Geometry: final body of the model. Coordinates: model frame, mm. Give positions to 0.01 mm unless a question says otherwise; leave off trailing zeros. Write each loop counter-clockwise with the first axis right and the second up, starting at its lowest first coordinate (ties: lowest second). Pieces come first, ordered by that corner, then holes.
Q1. Cut plane B-B on x = -64. Count the separate pieces of the cut face and the enclosed holes in it, plus the area to 3 significant figures.
Q2. Line query: L1, parallel to Y at x = -64, z = 5; L2, parallel to X at y = -174, z = 4.5; L3, parallel to X at y = -361.5, z = 7.75. Output: solid intervals per line, ascending.
Q3. Pin query (flat end, axial travel): pin 1 (8 mm diameter, centred on x = -13, y = -416.06, fed in from +Z). Return the tip coordinate at first contact, or that it passes through.
Q4. Cut plane A-A on x = -115.5. Return the cut outline in (y, z).
Q5. Cut plane C-C on y = -180.5. Return the cut outline in (x, z).
Q6. Draft query along Y for faces 1 (the face through (-34.045, -126.664, 4.056)), 2 (the face through (-65, -260, 0)), 3 (the face through (-10.69, -280.18, 4.06)), 4 (the face through (-113.568, -201.389, 3.944)). Return one class per face: pulls with the +Y half, pulls with the -Y half, needs draft (parallel to the pull), parting line crosses it, or undercut.
Autodesk Inventor part; units mm, degrees
ref_plane "Work Plane1" through (0, 0, 0) normal (0, 0, 1) x (1, 0, 0)
ref_plane "YZ Plane" through (0, 0, 0) normal (1, 0, 0) x (0, 1, 0)
ref_plane "XZ Plane" through (0, 0, 0) normal (0, 1, 0) x (-1, 0, 0)
ref_plane "Work Plane1" through (0, 0, 0) normal (0, 0, 1) x (1, 0, 0)
sketch "Sketch1" plane through (0, 0, 0) normal (0, 0, 1) x (1, 0, 0)
  line L0 (-65.5, -425.0611) -> (-65.5, -432.1593)
  line L1 (-120, -425.0611) -> (-65.5, -425.0611)
  ellipse E0 centre (-120, -417.963) end of major axis (-120, -425.0611) minor radius 4 (-124, -417.963) -> (-120, -425.0611) ccw
  line L2 (-124, -275.99) -> (-124, -417.963)
  ellipse E1 centre (-120, -275.99) end of major axis (-120, -268.8918) minor radius 4 (-123.8796, -274.2613) -> (-124, -275.99) ccw
  line L3 (-103.5409, -130.5299) -> (-123.8796, -274.2613)
  ellipse E2 centre (-99.6613, -132.2586) end of major axis (-99.6613, -125.1604) minor radius 4 (-103.1868, -128.9053) -> (-103.5409, -130.5299) ccw
  line L4 (-67.5255, -10.843) -> (-103.1868, -128.9053)
  ellipse E3 centre (-64, -14.1963) end of major axis (-64, -7.0982) minor radius 4 (-60.4745, -10.843) -> (-67.5255, -10.843) ccw
  line L5 (-24.8132, -128.9053) -> (-60.4745, -10.843)
  ellipse E4 centre (-28.3387, -132.2586) end of major axis (-28.3387, -125.1604) minor radius 4 (-24.4591, -130.5299) -> (-24.8132, -128.9053) ccw
  line L6 (-4.1204, -274.2613) -> (-24.4591, -130.5299)
  ellipse E5 centre (-8, -275.99) end of major axis (-8, -268.8918) minor radius 4 (-4, -275.99) -> (-4.1204, -274.2613) ccw
  line L7 (-4, -417.963) -> (-4, -275.99)
  ellipse E6 centre (-8, -417.963) end of major axis (-8, -425.0611) minor radius 4 (-8, -425.0611) -> (-4, -417.963) ccw
  line L8 (-62.5, -425.0611) -> (-8, -425.0611)
  line L9 (-62.5, -432.1593) -> (-62.5, -425.0611)
  line L10 (-8, -432.1593) -> (-62.5, -432.1593)
  ellipse E7 centre (-8, -417.963) end of major axis (-8, -432.1593) minor radius 8 (-8, -432.1593) -> (0, -417.963) ccw
  line L11 (0, -275.99) -> (0, -417.963)
  ellipse E8 centre (-8, -275.99) end of major axis (-8, -261.7937) minor radius 8 (0, -275.99) -> (-0.2409, -272.5326) ccw
  line L12 (-20.5796, -128.8012) -> (-0.2409, -272.5326)
  ellipse E9 centre (-28.3387, -132.2586) end of major axis (-28.3387, -118.0623) minor radius 8 (-20.5796, -128.8012) -> (-21.2877, -125.5519) ccw
  line L13 (-56.949, -7.4896) -> (-21.2877, -125.5519)
  ellipse E10 centre (-64, -14.1963) end of major axis (-64, 0) minor radius 8 (-56.949, -7.4896) -> (-71.051, -7.4896) ccw
  line L14 (-106.7123, -125.5519) -> (-71.051, -7.4896)
  ellipse E11 centre (-99.6613, -132.2586) end of major axis (-99.6613, -118.0623) minor radius 8 (-106.7123, -125.5519) -> (-107.4204, -128.8012) ccw
  line L15 (-127.7591, -272.5326) -> (-107.4204, -128.8012)
  ellipse E12 centre (-120, -275.99) end of major axis (-120, -261.7937) minor radius 8 (-127.7591, -272.5326) -> (-128, -275.99) ccw
  line L16 (-128, -417.963) -> (-128, -275.99)
  ellipse E13 centre (-120, -417.963) end of major axis (-120, -432.1593) minor radius 8 (-128, -417.963) -> (-120, -432.1593) ccw
  line L17 (-65.5, -432.1593) -> (-120, -432.1593)
  line L18 (-62.5, -425.0611) -> (-65.5, -425.0611)
  point P0 (0, 0)
extrude "Plate1" add sketch "Sketch1" along normal blind 8 contours L1 E0 L2 E1 L3 E2 L4 E3 L5 E4 L6 E5 L7 E6 L8 L18
sketch "Sketch2" plane through (0, 0, 8) normal (0, 0, 1) x (1, 0, 0)
  line L0 (-8, -425.0611) -> (-120, -425.0611)
  ellipse E0 centre (-8, -417.963) end of major axis (-8, -425.0611) minor radius 4 (-8, -425.0611) -> (-4, -417.963) ccw
  line L1 (-4, -275.99) -> (-4, -417.963)
  ellipse E1 centre (-8, -275.99) end of major axis (-8, -268.8918) minor radius 4 (-4, -275.99) -> (-4.1204, -274.2613) ccw
  line L2 (-24.4591, -130.5299) -> (-4.1204, -274.2613)
  ellipse E2 centre (-28.3387, -132.2586) end of major axis (-28.3387, -125.1604) minor radius 4 (-24.4591, -130.5299) -> (-24.8132, -128.9053) ccw
  line L3 (-60.4745, -10.843) -> (-24.8132, -128.9053)
  ellipse E3 centre (-64, -14.1963) end of major axis (-64, -7.0982) minor radius 4 (-60.4745, -10.843) -> (-67.5255, -10.843) ccw
  line L4 (-103.1868, -128.9053) -> (-67.5255, -10.843)
  ellipse E4 centre (-99.6613, -132.2586) end of major axis (-99.6613, -125.1604) minor radius 4 (-103.1868, -128.9053) -> (-103.5409, -130.5299) ccw
  line L5 (-123.8796, -274.2613) -> (-103.5409, -130.5299)
  ellipse E5 centre (-120, -275.99) end of major axis (-120, -268.8918) minor radius 4 (-123.8796, -274.2613) -> (-124, -275.99) ccw
  line L6 (-124, -417.963) -> (-124, -275.99)
  ellipse E6 centre (-120, -417.963) end of major axis (-120, -425.0611) minor radius 4 (-124, -417.963) -> (-120, -425.0611) ccw
  line L7 (-64, -470.7435) -> (-64, 33.682) construction
  line L8 (-8, -425.0611) -> (-120, -425.0611) construction
  circle A0 centre (-64, -365.0611) radius 11
  circle A1 centre (-64, -165.0611) radius 11
  circle A2 centre (-115, -416.0611) radius 5
  circle A3 centre (-115, -275.746) radius 5
  circle A4 centre (-94.6057, -131.6217) radius 5
  circle A5 centre (-64, -30.2968) radius 5
  circle A6 centre (-33.3943, -131.6217) radius 5
  circle A7 centre (-13, -275.746) radius 5
  circle A8 centre (-13, -416.0611) radius 5
  point P0 (0, 0)
  dimension "d1" = 22
  dimension "d2" = 22
  dimension "d3" = 10
  dimension "d4" = 10
  dimension "d5" = 10
  dimension "d7" = 10
  dimension "d9" = 10
  dimension "d11" = 10
  dimension "d13" = 10
  dimension "d15" = 9
  dimension "d16" = 9
  dimension "d17" = 4
  dimension "d18" = 9
  dimension "d19" = 9
  dimension "d20" = 9
  dimension "d21" = 9
  dimension "d22" = 9
  dimension "d23" = 9
  dimension "d24" = 9
  dimension "d25" = 9
  dimension "d26" = 9
  dimension "d27" = 9
  dimension "d28" = 9
  dimension "d29" = 9
  dimension "d30" = 60
  dimension "d31" = 60
  dimension "d33" = 200
extrude "zinkdrænshuller" cut sketch "Sketch2" against normal blind 8 contours A0 | A1 | A2 | A3 | A4 | A5 | A6 | A7 | A8
equation "\"d2\" = d1"
equation "\"d4\" = d3"
equation "\"d5\" = d6"
equation "\"d7\" = d8"
equation "\"d9\" = d10"
equation "\"d11\" = d12"
equation "\"d13\" = d14"
equation "\"d16\" = d15"
equation "\"d18\" = d16"
equation "\"d19\" = d16"
equation "\"d20\" = d16"
equation "\"d21\" = d16"
equation "\"d22\" = d16"
equation "\"d23\" = d16"
equation "\"d24\" = d16"
equation "\"d25\" = d16"
equation "\"d26\" = d16"
equation "\"d27\" = d16"
equation "\"d28\" = d16"
equation "\"d29\" = d16"
equation "\"d31\" = d30"
equation "\"d34\" = Thickness"
equation "\"d0\" = Thickness"
equation "\"BendRadius\" = Thickness"
equation "\"BendReliefWidth\" = Thickness"
equation "\"BendReliefDepth\" = 0.5 * Thickness"
equation "\"CornerReliefSize\" = 4 * Thickness"
equation "\"MinimumRemnant\" = 2 * Thickness"
equation "\"TransitionRadius\" = BendRadius"
equation "\"JacobiRadiusSize\" = BendRadius"
equation "\"GapSize\" = Thickness"
properties part number "bund vange-endeplade" material "S235JR"
Data:
1. separate pieces: 4
1. enclosed holes: 0
1. area: 2,910 mm2
2. L1: y = -425.06 to -376.06, -354.06 to -176.06, -154.06 to -35.3, -25.3 to -7.1
2. L2: x = -109.69 to -70.41, -57.59 to -18.31
2. L3: x = -124 to -74.41, -53.59 to -4
3. pin 1: passes through
4. outline: (-425.06, 0) - (-421.04, 0) - (-421.04, 8) - (-425.06, 8) - close; (-411.09, 0) - (-280.72, 0) - (-280.72, 8) - (-411.09, 8) - close; (-270.77, 0) - (-215.04, 0) - (-215.04, 8) - (-270.77, 8) - close
5. outline: (-110.61, 0) - (-17.39, 0) - (-17.39, 8) - (-110.61, 8) - close
6. face 1: undercut
6. face 2: needs draft
6. face 3: undercut
6. face 4: pulls with the +Y half
